from build123d import *

# Parameters (mm, degrees)
SKETCH_1_R               = 25.5
SKETCH_1_R_2             = 6
EXTRUDE_1_DEPTH          = 4
SKETCH_2_R               = 11.75
SKETCH_2_R_2             = 6
EXTRUDE_2_DEPTH          = 27.3
SKETCH_3_R               = 2.5
EXTRUDE_3_DEPTH          = 9
CUT_EXTRUDE_1_REACH      = 49.751
CUT_EXTRUDE_1_END_RADIUS = 11.75
SKETCH_5_R               = 3


with BuildPart() as part:
    # Эскиз1 → Бобышка-Вытянуть1 (new body)
    with BuildSketch(Plane(origin=(0, 0, 0), x_dir=(1, 0, 0), z_dir=(0, 1, 0))):
        with Locations(Location((0, 0, 0), (0, 0, 270))):
            Circle(SKETCH_1_R)
        with Locations(Location((0, 0, 0), (0, 0, 270))):
            Circle(SKETCH_1_R_2, mode=Mode.SUBTRACT)
    extrude(amount=EXTRUDE_1_DEPTH)

    # Эскиз2 → Бобышка-Вытянуть2 (add)
    with BuildSketch(Plane(origin=(0, 4, 0), x_dir=(1, 0, 0), z_dir=(0, 1, 0))):
        with Locations(Location((0, 0, 0), (0, 0, 270))):
            Circle(SKETCH_2_R)
        with Locations(Location((0, 0, 0), (0, 0, 270))):
            Circle(SKETCH_2_R_2, mode=Mode.SUBTRACT)
    extrude(amount=EXTRUDE_2_DEPTH)

    # Эскиз3 → Бобышка-Вытянуть3 (add)
    with BuildSketch(Plane.XZ):
        with Locations(Location((-17.5, 0, 0), (0, 0, 90))):
            Circle(SKETCH_3_R)
        with Locations(Location((17.5, 0, 0), (0, 0, 90))):
            Circle(SKETCH_3_R)
    extrude(amount=EXTRUDE_3_DEPTH)

    # Вырез-Вытянуть1: up to this cylinder (the profile starts inside it)
    cut_extrude_1_end = Plane(origin=(0, 21.3, 0), z_dir=(0, -1, 0)) * Cylinder(CUT_EXTRUDE_1_END_RADIUS, 124.002, mode=Mode.PRIVATE)
    # Эскиз5 → Вырез-Вытянуть1 (cut, up to the surface)
    with BuildSketch(Plane.XY, mode=Mode.PRIVATE) as cut_extrude_1_sk1:
        with Locations((0, 21.3)):
            Circle(SKETCH_5_R)
    cut_extrude_1_tool1 = extrude(cut_extrude_1_sk1.sketch, amount=-CUT_EXTRUDE_1_REACH, mode=Mode.PRIVATE) & cut_extrude_1_end
    add(cut_extrude_1_tool1.solids().sort_by_distance((0, 21.3, 0))[0], mode=Mode.SUBTRACT)


solid = part.part
Verification items for the finished model (mm, model axes). A direction names the side the tool comes from. Give positions to 0.01 mm unless a question says otherwise; leave off trailing zeros. Loops run counter-clockwise (first coordinate to the right, second up) from the corner with the lowest first, then second, coordinate; pieces in that order, holes last.
1) Sectioned sample at D-D, the plane x = 18.5. Enter the section's corners in (y, z).
2) Sectioned sample at B-B, the plane y = -6. Enter the section's corners in (x, z).
3) Sectioned sample at A-A, the plane z = 0. Enter the section's corners in (x, y).
4) Draft check along X on faces 1 (the cylindrical face through (-20, -4, 0)), 2 (the flat face through (-18, -9, 0)), 3 (the cylindrical face through (-24.9, 2, -5.5)). Enter one of: pulls with the +X half, pulls with the -X half, needs draft (parallel to the pull), parting line crosses it, or undercut.
5) Set-up check for faces 4 (the flat face through (17, -9, 0)), 5 (the flat face through (-5, 31.3, 5)), 6 (the flat face through (-5, 4, 11)), 7 (the cylindrical face through (1.384, 18.638, -8.428)), 8 (the cylindrical face through (19.94, -4.44, -0.54)): record each of +Z, -Z, +X, -X, +Y, -Y from which the full face is reachable in a straight line by a thin tool's end or side.
6) Thickness scan on line 1 along X through (y, z) = (24.5, 0); line 2 along Y through (x, z) = (15.5, -10). Record the ranges inside material, lowest first.
7) Sectioned sample at C-C, the plane y = 1. Enter the section's corners in (x, z).
8) Depth check by flat-ended pin: pin 1 Ø5 at (x, z) = (-6, -17.5) entering from +Y; pin 2 Ø6 at (x, y) = (-1.5, -3.5) entering from +Z; pin 3 Ø6 at (x, y) = (7, 20) entering from +Z; pin 4 Ø2 at (x, z) = (9, -14.5) entering from -Y. Enter the tip coordinate at first touch or a pass-through.
Answers:
1. outline: (-9, -2.29) - (0, -2.29) - (0, -17.55) - (4, -17.55) - (4, 17.55) - (0, 17.55) - (0, 2.29) - (-9, 2.29) - close
2. outline: circle Ø5 at (-17.5, 0); circle Ø5 at (17.5, 0)
3. outline: (-25.5, 0) - (-20, 0) - (-20, -9) - (-15, -9) - (-15, 0) - (-6, 0) - (-6, 31.3) - (-11.75, 31.3) - (-11.75, 4) - (-25.5, 4) - close; (6, 0) - (15, 0) - (15, -9) - (20, -9) - (20, 0) - (25.5, 0) - (25.5, 4) - (11.75, 4) - (11.75, 31.3) - (6, 31.3) - close
4. face 1: undercut
4. face 2: needs draft
4. face 3: parting line crosses it
5. face 4: +Z, -Z, +X, -X, -Y
5. face 5: +Z, -Z, +X, -X, +Y
5. face 6: +Y
5. face 7: -Z
5. face 8: -Y
6. line 1: x = -11.75 to -6, 6 to 11.75
6. line 2: y = 0 to 4
7. outline: circle Ø51 at (0, 0); hole circle Ø12 at (0, 0)
8. pin 1: stops at y = 4
8. pin 2: passes through
8. pin 3: stops at z = 11.05
8. pin 4: stops at y = 0
